For this review, take the finished solid that the model builds, in its own axes (mm). A direction names the side the tool comes from. Give positions to 0.01 mm unless a question says otherwise; leave off trailing zeros. Order: outer loops, then holes, each group sorted by start corner. A loop starts at its lowest first (then second) coordinate and runs counter-clockwise, first axis right, second up.
Item 1: Consider section D-D (y = 1.5). Give the boundary of the cut face in (x, z), plus the area to 3 significant figures.
Item 2: Consider section C-C (y = 6). Give the boundary of the cut face in (x, z), plus the area to 3 significant figures.
Item 3: For probe 1 along Y at (x, z) = (0.2, 0.9); probe 2 along Y at (x, z) = (0.5, -1.4); probe 3 along Z at (x, y) = (-0.05, 1.25), list the stretches that pass through material, from the lowest coordinate up.
Item 4: Consider section A-A (z = 0). Give the boundary of the cut face in (x, y), plus the area to 3 significant figures.
Item 5: Consider section B-B (x = 0). Give the boundary of the cut face in (y, z).
Item 6: For P1, Ø2, axis at y = 4, z = -2, coming from the +X side; P2, Ø1.5, axis at x = 1, z = 1.5, coming from the -Y side; P3, Ø0.5, axis at x = 0, z = -0.5, coming from the +Y side, all flat-tipped, find the tip position at first contact; note any pin that passes through.
Item 7: Machinability: for faces 1 (the flat face through (1, 2, 0)), 2 (the flat face through (-0.3, 6, 0)), 3 (the flat face through (0, 0, 0)), which of the approach directions +Z, -Z, +X, -X, +Y, -Y give a long, thin tool a straight path to every point of the face, cutting with its end or side? Answer none if there is none.
```python
from build123d import *

# Parameters (mm, degrees)
SKETCH1_R               = 2.5
BOSS_EXTRUDE1_DEPTH     = 6.7
SKETCH2_OUTSIDE_W       = 8.948
SKETCH2_OUTSIDE_H       = 8.948
SKETCH2_OUTSIDE_R       = 0.85
CUT_EXTRUDE1_DEPTH      = 2
SKETCH3_OUTSIDE_W       = 8.948
SKETCH3_OUTSIDE_H       = 8.948
SKETCH3_OUTSIDE_R       = 1.25
CUT_EXTRUDE2_DEPTH      = 2.85
CHAMFER1_SIZE           = 0.2
CUT_EXTRUDE3_DEPTH      = 8.575618787
CUT_EXTRUDE3_DEPTH_BACK = 8.575618787
SKETCH4_W               = 0.6
SKETCH4_H               = 0.9
CHAMFER2_SIZE           = 0.25


with BuildPart() as part:
    # Sketch1 → Boss-Extrude1 (new body)
    with BuildSketch(Plane(origin=(0, 0, 0), x_dir=(1, 0, 0), z_dir=(0, 1, 0))):
        with Locations(Location((0, 0, 0), (0, 0, 270))):
            Circle(SKETCH1_R)
    extrude(amount=BOSS_EXTRUDE1_DEPTH)

    # Sketch2 outside → Cut-Extrude1 (cut)
    with BuildSketch(Plane.XZ):
        Rectangle(SKETCH2_OUTSIDE_W, SKETCH2_OUTSIDE_H)
        with Locations(Location((0, 0, 0), (0, 0, 270))):
            Circle(SKETCH2_OUTSIDE_R, mode=Mode.SUBTRACT)
    extrude(amount=-CUT_EXTRUDE1_DEPTH, mode=Mode.SUBTRACT)

    # Sketch3 outside → Cut-Extrude2 (cut)
    with BuildSketch(Plane.XZ.offset(-2)):
        Rectangle(SKETCH3_OUTSIDE_W, SKETCH3_OUTSIDE_H)
        with Locations(Location((0, 0, 0), (0, 0, 270))):
            Circle(SKETCH3_OUTSIDE_R, mode=Mode.SUBTRACT)
    extrude(amount=-CUT_EXTRUDE2_DEPTH, mode=Mode.SUBTRACT)

    # Chamfer1
    chamfer1_edges = [part.edges().sort_by_distance(p)[0] for p in [
        (0, 6.7, -2.5),
    ]]
    chamfer(chamfer1_edges, length=CHAMFER1_SIZE)

    # Sketch4 → Cut-Extrude3 (cut, two sides: drawn at the far end of the back side and taken through both)
    with BuildSketch(Plane.XY.offset(-CUT_EXTRUDE3_DEPTH_BACK)):
        with Locations((0, 6.25)):
            Rectangle(SKETCH4_W, SKETCH4_H)
    extrude(amount=CUT_EXTRUDE3_DEPTH + CUT_EXTRUDE3_DEPTH_BACK, mode=Mode.SUBTRACT)

    # Chamfer2
    chamfer2_edges = [part.edges().sort_by_distance(p)[0] for p in [
        (0, 0, 0.85),
    ]]
    chamfer(chamfer2_edges, length=CHAMFER2_SIZE)


solid = part.part
```
Resolved:
1. outline: circle Ø1.7 at (0, 0)
1. area: 2.27 mm2
2. outline: (-0.3, -2.48) - (-0.3, 2.48) arc R2.5 ccw to start; (0.3, -2.48) arc R2.5 ccw to (0.3, 2.48) - close
2. area: 16.6 mm2
3. probe 1: y = 2 to 5.8
3. probe 2: y = 4.85 to 6.7
3. probe 3: z = -0.85 to 0.85
4. outline: (-2.5, 4.85) - (-1.25, 4.85) - (-1.25, 2) - (-0.85, 2) - (-0.85, 0.25) - (-0.6, 0) - (0.6, 0) - (0.85, 0.25) - (0.85, 2) - (1.25, 2) - (1.25, 4.85) - (2.5, 4.85) - (2.5, 6.5) - (2.3, 6.7) - (0.3, 6.7) - (0.3, 5.8) - (-0.3, 5.8) - (-0.3, 6.7) - (-2.3, 6.7) - (-2.5, 6.5) - close
4. area: 19.1 mm2
5. outline: (0, -0.6) - (0.25, -0.85) - (2, -0.85) - (2, -1.25) - (4.85, -1.25) - (4.85, -2.5) - (5.8, -2.5) - (5.8, 2.5) - (4.85, 2.5) - (4.85, 1.25) - (2, 1.25) - (2, 0.85) - (0.25, 0.85) - (0, 0.6) - close
6. P1: stops at x = 2.02
6. P2: stops at y = 2
6. P3: stops at y = 5.8
7. face 1: -Y
7. face 2: +Z, -Z, +Y
7. face 3: +Z, -Z, +X, -X, -Y
